Answer from the drawing. Dimensions are ordinates in mm from the lowest x, y and z of the part. A direction names the side the tool comes from. Give positions to 0.01 mm unless a question says otherwise; leave off trailing zeros. Loops run counter-clockwise (first coordinate to the right, second up) from the corner with the lowest first, then second, coordinate; pieces in that order, holes last. Notation, with made-up numbers: (9, -35.5) - (56, -35.5) arc R15 ccw to (56, -18.5) - close; hole circle Ø7 at (-12.5, 10.5). An arc over 180 degrees is marked (long way). Write each question's results on one line, items separated by ' | '. Start each with the question number.
Q1. Find the intervals of material crossed by line 1 (Z direction, x = 6, y = 0.75); line 2 (Z direction, x = 14.5, y = 2), in increasing order. Write a range as from..to.
Q2. For the marked faces 4, 5, 6, 7 and 8, determine the directions among +Z, -Z, +X, -X, +Y, -Y from which every point of the face is accessible in a straight line to the end or side of a thin tool.
Q3. The part is cut by section C-C, the plane z = 20. Write down the section's boundary in (x, y).
Q4. Given pin 1 (3.5 mm diameter, centred on x = 12.5, y = 7, fed in from -Z); pin 2 (4.5 mm diameter, centred on y = 7, z = 10.5, fed in from -X); pin 3 (4.5 mm diameter, centred on y = 7, z = 16.5, fed in from +X), each flat-ended and moving along its own axis, determine where each tip first touches the part or whether it passes through.
Q5. Determine the mould class of the marked faces 1, 2 and 3 for opening direction Y: +Y half, -Y half, draft (parallel to the pull), parting line (faces both ways), or undercut.
Q6. The part is cut by section D-D, the plane z = 29.5. Write down the section's boundary in (x, y), plus the area to 3 significant figures.
Q7. The part is cut by section B-B, the plane y = 2.2. Write down the section's boundary in (x, z), plus the area to 3 significant figures.
Q8. The part is cut by section A-A, the plane x = 13.5. Write down the section's boundary in (y, z).
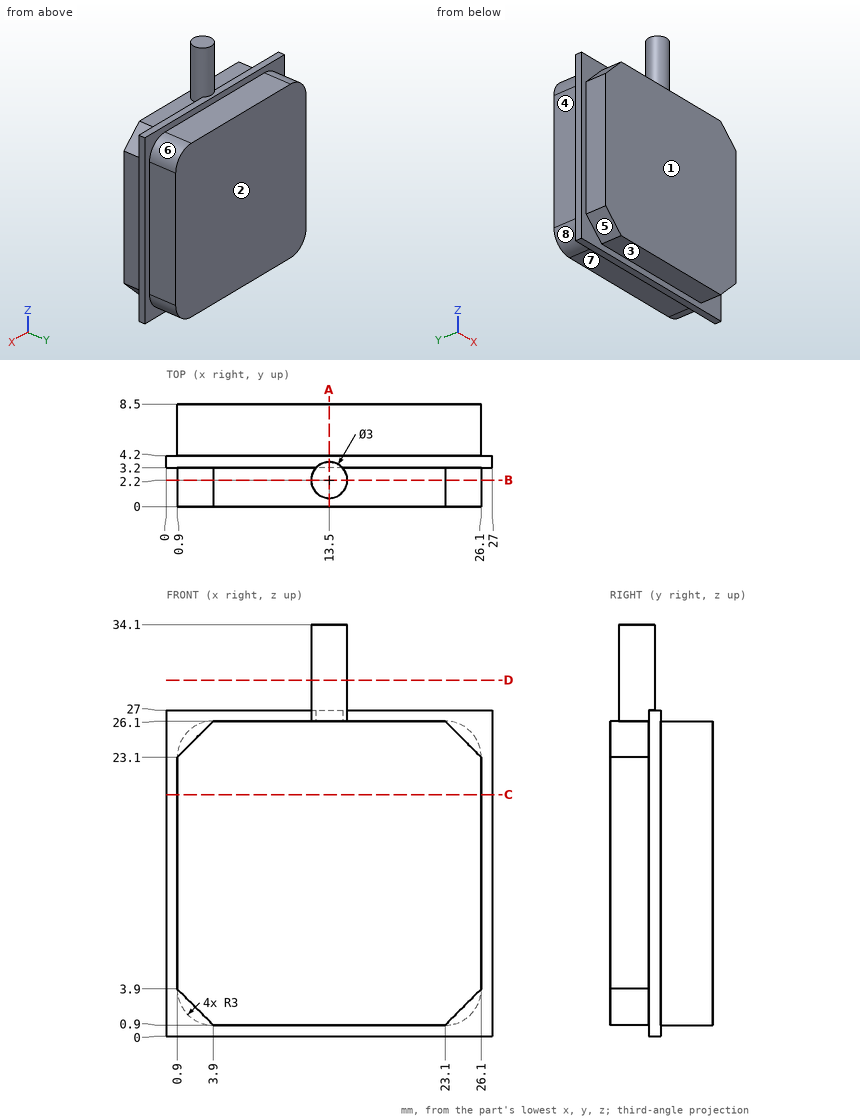
Check sheet entries:
1) line 1: z = 0.9..26.1 | line 2: z = 0.9..34.1
2) face 4: +Z, -Z, -X, +Y | face 5: -Z, -X, -Y | face 6: +Z, +X, +Y | face 7: -Z, +X, -X, +Y | face 8: -Z, -X, +Y
3) outline: (0, 3.2) - (0.9, 3.2) - (0.9, 0) - (26.1, 0) - (26.1, 3.2) - (27, 3.2) - (27, 4.2) - (26.1, 4.2) - (26.1, 8.5) - (0.9, 8.5) - (0.9, 4.2) - (0, 4.2) - close
4) pin 1: stops at z = 0.9 | pin 2: stops at x = 0.9 | pin 3: stops at x = 26.1
5) face 1: -Y half | face 2: +Y half | face 3: draft
6) outline: circle Ø3 at (13.5, 2.2) | area: 7.07 mm^2
7) outline: (0.9, 3.9) - (3.9, 0.9) - (23.1, 0.9) - (26.1, 3.9) - (26.1, 23.1) - (23.1, 26.1) - (15, 26.1) - (15, 34.1) - (12, 34.1) - (12, 26.1) - (3.9, 26.1) - (0.9, 23.1) - close | area: 641 mm^2
8) outline: (0, 0.9) - (3.2, 0.9) - (3.2, 0) - (4.2, 0) - (4.2, 0.9) - (8.5, 0.9) - (8.5, 26.1) - (4.2, 26.1) - (4.2, 27) - (3.7, 27) - (3.7, 34.1) - (0.7, 34.1) - (0.7, 26.1) - (0, 26.1) - close
